Read the model definition and answer for the solid it produces. Units are mm, in the model's axes. Face numbers are marked on the shaded views. A direction names the side the tool comes from. Give positions to 0.01 mm unless a question says otherwise; leave off trailing zeros. Write each loop counter-clockwise with the first axis right and the second up, starting at its lowest first coordinate (ties: lowest second). Pieces come first, ordered by that corner, then holes. Notation, with made-up numbers: M -15.75,55.5 L 13.25,55.5 A25 ccw 13.25,92.5 Z; hole C 65.5,-0.75 d6. An arc over 180 degrees is marked long. Put each result on its own line as item: value.
from build123d import *

# Parameters (mm, degrees)
F1_DEPTH  = 25
F2_DEPTH  = 15
F2_FACE_W = 15
F2_FACE_H = 25
F3_DEPTH  = 10


with BuildPart() as f1:
    # F0 (on Front) → F1 (new body, symmetric)
    with BuildSketch(Plane.XZ):
        Polygon((-25, 22.5), (-25, -22.5), (25, -22.5), (25, 22.5), (-13, 22.5), align=None)
    extrude(amount=F1_DEPTH, both=True)

    # F0 (on Front) → F2 (join)
    with BuildSketch(Plane.XZ):
        Polygon((-25, 22.5), (-25, -22.5), (25, -22.5), (25, 22.5), (-13, 22.5), align=None)
        with BuildLine():
            ThreePointArc((16.44358, 62.473942), (-12.769199, 51.29013), (-25, 22.5))
            Line((-25, 22.5), (-13, 22.5))
            ThreePointArc((-13, 22.5), (-4.281853, 42.802959), (16.44358, 50.462762))
            Line((16.44358, 50.462762), (16.44358, 62.473942))
        make_face()
        Polygon((36.44358, 62.473942), (16.44358, 62.473942), (16.44358, 50.462762), (16.44358, 37.473942), (36.44358, 37.473942), align=None)
    extrude(amount=F2_DEPTH)

    # F2_face (on face) → F3 (join)
    with BuildSketch(Plane(origin=(36.44358, -7.5, 49.973942), x_dir=(0, 1, 0), z_dir=(1, 0, 0))):
        Rectangle(F2_FACE_W, F2_FACE_H)
    extrude(amount=F3_DEPTH)


solid = f1.part
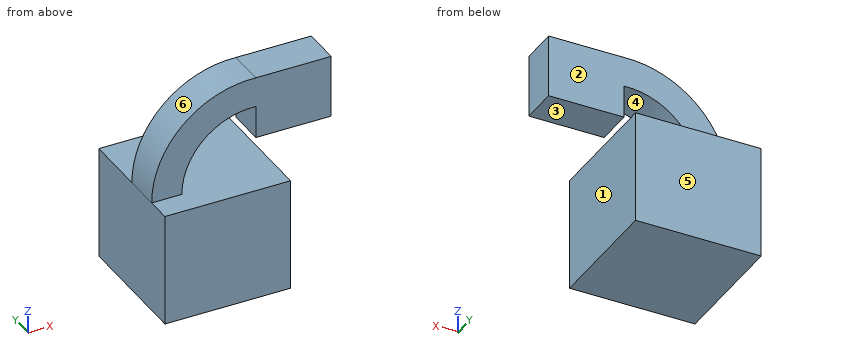
(1) For a pull along Z with two mould halves and no side action, classify the marked faces 4, 5 and 6 as +Z half, -Z half, draft (parallel to the pull), parting line (faces both ways), or undercut.
Result:
face 4: undercut
face 5: draft
face 6: +Z half
(2) Section A-A on x = 7 is taken. Determine the outline of the cut face in (y, z).
Result:
outline: M -25,-22.5 L 25,-22.5 L 25,22.5 L -25,22.5 Z; M -15,49.33 L 0,49.33 L 0,61.69 L -15,61.69 Z
(3) Straight lines are drawn through the part: line 1 along Z through (x, y) = (23.5, -5); line 2 along X through (y, z) = (-22, -12); line 3 along Z through (x, y) = (38.5, -12.5). For each, find the intervals that lie inside material, in ascending order. Write a range as from..to.
Result:
line 1: z = -22.5..22.5, 37.47..62.47
line 2: x = -25..25
line 3: z = 37.47..62.47
(4) Given pin 1 Ø5 at (x, y) = (-10, -9.5) entering from +Z; pin 2 Ø3 at (x, z) = (-16, 43) entering from -Y; pin 3 Ø25 at (x, y) = (-3, 11.5) entering from +Z, each flat-ended and moving along its own axis, determine where each tip first touches the part or whether it passes through.
Result:
pin 1: stops at z = 55.57
pin 2: stops at y = -15
pin 3: stops at z = 60.29
(5) Section B-B on x = 42 is taken. Determine the outline of the cut face in (y, z), and give its area (3 significant figures).
Result:
outline: M -15,37.47 L 0,37.47 L 0,62.47 L -15,62.47 Z
area: 375 mm²
(6) Section D-D on x = -6.5 is taken. Determine the outline of the cut face in (y, z), and give its area (3 significant figures).
Result:
outline: M -25,-22.5 L 25,-22.5 L 25,22.5 L -25,22.5 Z; M -15,40.44 L 0,40.44 L 0,56.23 L -15,56.23 Z
area: 2,490 mm²
(7) Section C-C on y = 5 is taken. Determine the outline of the cut face in (x, z), and give its area (3 significant figures).
Result:
outline: M -25,-22.5 L 25,-22.5 L 25,22.5 L -25,22.5 Z
area: 2,250 mm²
(8) Which of the six approach directions +Z, -Z, +X, -X, +Y, -Y give full straight-line access (tool end or side, diameter ignored) to the marked faces 1, 2 and 3?
Result:
face 1: -Z, +X, +Y, -Y
face 2: +Z, +X, -X, +Y
face 3: +X, +Y, -Y
